```python
from build123d import *

# Parameters (mm, degrees)
BOSS_EXTRUDE1_DEPTH      = 5.999999938
SKETCH3_R                = 9
CUT_EXTRUDE1_DEPTH       = 3
CUT_EXTRUDE5_DEPTH       = 1
CUT_EXTRUDE5_DEPTH_BACK  = 3
EXTRUDE_THIN3_DEPTH      = 5.999999938
CUT_EXTRUDE9_DEPTH       = 1
CUT_EXTRUDE10_DEPTH      = 1
CUT_EXTRUDE10_DEPTH_BACK = 1
BOSS_EXTRUDE3_DEPTH      = 9
BOSS_EXTRUDE3_DRAFT      = 3
SKETCH14_R               = 8
CUT_EXTRUDE13_DEPTH      = 2.5
CUT_EXTRUDE15_DEPTH      = 10
CUT_EXTRUDE15_DEPTH_BACK = 1.000000032


with BuildPart() as part:
    # Sketch2 → Boss-Extrude1 (new body)
    with BuildSketch(Plane(origin=(0, 0, 0), x_dir=(1, 0, 0), z_dir=(0, 1, 0))):
        with BuildLine():
            Line((0, 0), (60, 0))
            ThreePointArc((60, 0), (76.794228634, 4.5), (60, 9))
            Line((60, 9), (0, 9))
            Line((0, 9), (0, 0))
        make_face()
    extrude(amount=BOSS_EXTRUDE1_DEPTH)

    # Sketch3 → Cut-Extrude1 (cut)
    with BuildSketch(Plane(origin=(0, 5.999999938, 0), x_dir=(1, 0, 0), z_dir=(0, 1, 0))):
        with Locations((67.794228634, 4.5)):
            Circle(SKETCH3_R)
    extrude(amount=-CUT_EXTRUDE1_DEPTH, mode=Mode.SUBTRACT)

    # Sketch5 → Cut-Extrude5 (cut, two sides)
    with BuildSketch(Plane(origin=(0, 5.999999938, 0), x_dir=(1, 0, 0), z_dir=(0, 1, 0))) as cut_extrude5_sk:
        with BuildLine():
            Line((141.885159374, -104.803724525), (60, 0))
            ThreePointArc((60, 0), (57.540129042, 4.245085458), (56.330788983, 9))
            Line((56.330788983, 9), (41.599359793, 141.181636372))
            Line((41.599359793, 141.181636372), (287.915588972, 241.602327681))
            Line((287.915588972, 241.602327681), (388.201388554, -4.383033215))
            Line((388.201388554, -4.383033215), (141.885159374, -104.803724525))
        make_face()
    extrude(amount=CUT_EXTRUDE5_DEPTH, mode=Mode.SUBTRACT)
    extrude(cut_extrude5_sk.sketch, amount=-CUT_EXTRUDE5_DEPTH_BACK, mode=Mode.SUBTRACT)

    # Sketch6 → Extrude-Thin3 (add)
    with BuildSketch(Plane(origin=(0, 5.999999938, 0), x_dir=(1, 0, 0), z_dir=(0, 1, 0))):
        with BuildLine():
            ThreePointArc((2.566768688, 3.148851961), (-7.252946342, 4.805124242), (2.704294257, 4.958097373))
            Line((2.704294257, 4.958097373), (0.178709714, 4.68787022))
            ThreePointArc((0.178709714, 4.68787022), (-4.720252661, 4.61260744), (0.111047134, 3.797721478))
            Line((0.111047134, 3.797721478), (2.566768688, 3.148851961))
        make_face()
    extrude(amount=-EXTRUDE_THIN3_DEPTH)

    # Sketch7 → Cut-Extrude9 (cut)
    with BuildSketch(Plane(origin=(0, 5.999999938, 0), x_dir=(1, 0, 0), z_dir=(0, 1, 0))):
        Polygon((0, 0), (0, 9), (10.83654063, 0), align=None)
    extrude(amount=-CUT_EXTRUDE9_DEPTH, mode=Mode.SUBTRACT)

    # Sketch8 → Cut-Extrude10 (cut, two sides)
    with BuildSketch(Plane(origin=(0, 5.999999938, 0), x_dir=(1, 0, 0), z_dir=(0, 1, 0))) as cut_extrude10_sk:
        Polygon((0, 9), (1.982929041, 7.353131135), (3.117751909, 9), align=None)
    extrude(amount=CUT_EXTRUDE10_DEPTH, mode=Mode.SUBTRACT)
    extrude(cut_extrude10_sk.sketch, amount=-CUT_EXTRUDE10_DEPTH_BACK, mode=Mode.SUBTRACT)


with BuildPart() as boss_extrude3_tool:
    # Sketch9 → Boss-Extrude3 (with draft: the straight prism first)
    with BuildSketch(Plane(origin=(0, 0, 0), x_dir=(-1, 0, 0), z_dir=(0, -1, 0))):
        with BuildLine():
            Line((-73.720761097, -2.273198134), (-69.720761097, -2.273198134))
            ThreePointArc((-69.720761097, -2.273198134), (-72.492846156, 0.552836778), (-72.794228634, 4.5))
            Line((-72.794228634, 4.5), (-76.794228634, 4.5))
            ThreePointArc((-76.794228634, 4.5), (-75.989922386, 0.781048008), (-73.720761097, -2.273198134))
        make_face()
    extrude(amount=BOSS_EXTRUDE3_DEPTH)
    # Boss-Extrude3: the draft: its side faces are tilted about the plane it starts from
    boss_extrude3_sides = [boss_extrude3_tool.faces().sort_by_distance(p)[0] for p in [
        (72.492846156, -4.5, -0.552836778),
        (74.794228634, -4.5, -4.5),
        (75.989922386, -4.5, -0.781048008),
        (71.720761097, -4.5, 2.273198134),
    ]]
    draft(boss_extrude3_sides, Plane(origin=(0, 0, 0), x_dir=(-1, 0, 0), z_dir=(0, -1, 0)), BOSS_EXTRUDE3_DRAFT)


with BuildPart() as part_1:
    add(part.part)

    # Boss-Extrude3: add boss_extrude3_tool
    add(boss_extrude3_tool.part)

    # Sketch14 → Cut-Extrude13 (cut)
    with BuildSketch(Plane(origin=(0, 2.999999938, 0), x_dir=(1, 0, 0), z_dir=(0, 1, 0))):
        with Locations((67.794228634, 4.5)):
            Circle(SKETCH14_R)
    extrude(amount=-CUT_EXTRUDE13_DEPTH, mode=Mode.SUBTRACT)

    # Sketch16 → Cut-Extrude15 (cut, two sides)
    with BuildSketch(Plane(origin=(0, 0, 0), x_dir=(-1, 0, 0), z_dir=(0, -1, 0))) as cut_extrude15_sk:
        Polygon((129.561472715, 112.505246853), (0, 8.882522618), (-11.105987806, 0), (-140.667460521, -103.622724235), (66.57798795, -362.745669665), (336.806921186, -146.617698577), align=None)
    extrude(amount=CUT_EXTRUDE15_DEPTH, mode=Mode.SUBTRACT)
    extrude(cut_extrude15_sk.sketch, amount=-CUT_EXTRUDE15_DEPTH_BACK, mode=Mode.SUBTRACT)


solid = part_1.part
```
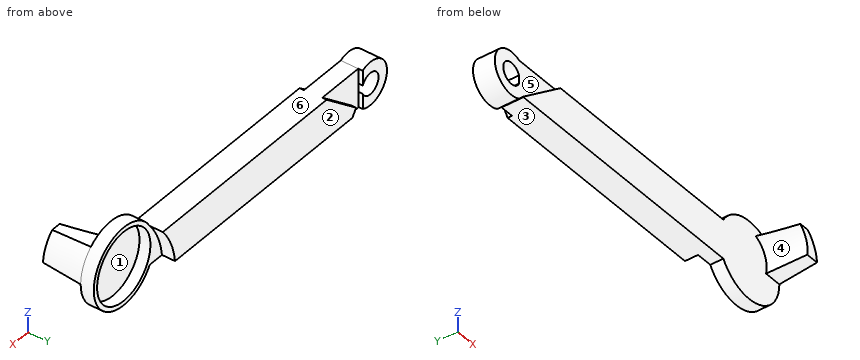
Can you work these out from the model? Positions are in its coordinate system, mm. Face numbers are marked on the shaded views. A direction names the side the tool comes from. Round coordinates to 2 decimals unless told otherwise and drop trailing zeros. Loops run counter-clockwise (first coordinate to the right, second up) from the corner with the lowest first, then second, coordinate; pieces in that order, holes last. Notation, with made-up numbers: M -0.75,46.5 L 54.25,46.5 A27 ccw 54.25,69.5 Z; hole C 41,-32.5 d5. An arc over 180 degrees is marked long. Answer in a Markdown table with one row per item.
1. Thinking about a two-plate mould opening in Z: for the marked faces 3, 4, 5 and 6, which applies, pulls with the +Z half, pulls with the -Z half, needs draft (parallel to the pull), parting line crosses it, or undercut?
Established:
| item | result |
|---|---|
| face 3 | pulls with the -Z half |
| face 4 | undercut |
| face 5 | needs draft |
| face 6 | pulls with the +Z half |
2. If we section it at D-D, the plane x = 67: Please give me the cut outline in (y, z), plus the area to 3 significant figures.
Established:
| item | result |
|---|---|
| outline | M 0,-13.46 L 3,-13.46 L 3,-12.46 L 0.5,-12.46 L 0.5,3.46 L 3,3.46 L 3,4.46 L 0,4.46 Z |
| area | 14.0 mm² |
3. Please list where these lines run through material, in increasing order: line 1 (X direction, y = 1.1, z = -4.5); line 2 (Z direction, x = 50, y = 1); line 3 (Y direction, x = 59, z = -4). Write a range as from..to.
Established:
| item | result |
|---|---|
| line 1 | -7.27..-4.73, 0..59.79, 75.79..76.79 |
| line 2 | -9..0 |
| line 3 | 0..3 |
4. If we section it at B-B, the plane x = 30.5: Please give me the cut outline in (y, z), plus the area to 3 significant figures.
Established:
| item | result |
|---|---|
| outline | M 0,-9 L 6,-9 L 6,0 L 0,0 Z |
| area | 54.0 mm² |
5. If we section it at C-C, the plane y = -6.25: Please give me the cut outline in (x, z), plus the area to 3 significant figures.
Established:
| item | result |
|---|---|
| outline | M 70.89,1.95 A6.1 cw 73.21,-4.17 L 76.46,-4.17 A8.67 ccw 73.6,1.95 Z |
| area | 17.1 mm² |
6. I'm going to push flat-ended pins straight in: pin 1 Ø3 at (x, z) = (-2.27, -4.43) entering from -Y; pin 2 Ø5 at (x, y) = (23, 1.5) entering from +Z; pin 3 Ø9 at (x, z) = (63, -4) entering from +Y; pin 4 Ø3 at (x, z) = (30, -7.5) entering from -Y. Where does each tip first touch, or does it pass through?
Established:
| item | result |
|---|---|
| pin 1 | through |
| pin 2 | z = 0 |
| pin 3 | y = 3 |
| pin 4 | y = 0 |
7. On a 3-axis mill with a long thin cutter (end or side, diameter ignored), from which of +Z, -Z, +X, -X, +Y, -Y can I reach the whole of each face in a straight line? I mean the marked faces 1 and 2. Say none if no direction works.
Established:
| item | result |
|---|---|
| face 1 | +Y |
| face 2 | +Z, -Z, +X, -X, +Y |
8. If we section it at A-A, the plane x = -2: Please give me the cut outline in (y, z), plus the area to 3 significant figures.
Established:
| item | result |
|---|---|
| outline | M 1,-9.42 L 6,-9.42 L 6,-6.87 L 1,-6.87 Z; M 1,-1.98 L 6,-1.98 L 6,0.57 L 1,0.57 Z |
| area | 25.5 mm² |
